Part model, mm, in its own coordinate system. A direction names the side the tool comes from. Round coordinates to 2 decimals unless told otherwise and drop trailing zeros. Loops run counter-clockwise (first coordinate to the right, second up) from the corner with the lowest first, then second, coordinate; pieces in that order, holes last. Notation, with made-up numbers: M 50.5,-34.75 L 98.5,-34.75 A14 cw 98.5,-20.75 Z; hole C -31.5,60.25 d4. An arc over 180 degrees is marked long. Put each result on its own line as item: value. Start each with the question number.
1) Slice it at B-B on z = 0. Give the cut face in (x, y).
2) Slice it at D-D on y = 34. Give the cut face in (x, z).
3) Probe line 1 along Y through (x, z) = (48.95, 9); line 2 along X through (y, z) = (42.5, 0); line 3 along Z through (x, y) = (21, 56). List the from-to ranges inside material, lowest first.
4) Slice it at A-A on y = 13.27. Give the cut face in (x, z), then the cut area to 3 significant figures.
5) Drop flat-ended pins along their axis: pin 1 Ø6.5 at (y, z) = (38.5, 9.5) entering from -X; pin 2 Ø8 at (x, y) = (-5.5, 7) entering from +Z. Give the stop position or say it passes through.
6) Pull direction X, two halves, no side cores. Call faces 4 (the flat face through (-1, 0, -2)), 5 (the flat face through (47, 38, 9)), 6 (the cylindrical face through (-47.464, 33.736, -0.325)): +X half, -X half, draft (parallel to the pull), parting line (faces both ways), or undercut.
7) Slice it at C-C on x = -46. Give the cut face in (y, z), then the cut area to 3 significant figures.
8) Which spindle directions (+Z, -Z, +X, -X, +Y, -Y) get a long thin tool onto all of the face, cutting with end or side? Do faces 1 (the flat face through (3.5, 10, 4.6)), 2 (the flat face through (50, 33, 4)), 3 (the flat face through (-2, 38, 5)). Say none if no direction does.
```python
from build123d import *

# Parameters (mm, degrees)
SKETCH1_W           = 100
SKETCH1_H           = 10
BOSS_EXTRUDE1_DEPTH = 66.54
CUT_EXTRUDE1_REACH  = 85.382
SKETCH2_R           = 1.5
LPATTERN1_COUNT     = 2
LPATTERN1_PITCH     = 92
SKETCH3_W           = 100
SKETCH3_H           = 10
CUT_EXTRUDE2_DEPTH  = 3
SKETCH4_W           = 3
SKETCH4_H           = 56.54
BOSS_EXTRUDE2_DEPTH = 8
CUT_EXTRUDE3_REACH  = 122.816
SKETCH5_R           = 1.5


with BuildPart() as part:
    # Sketch1 → Boss-Extrude1 (new body)
    with BuildSketch(Plane(origin=(0, 0, 0), x_dir=(1, 0, 0), z_dir=(0, 1, 0))):
        Rectangle(SKETCH1_W, SKETCH1_H)
    extrude(amount=BOSS_EXTRUDE1_DEPTH)

    # Sketch2 → Cut-Extrude1 (cut, up to next)
    with BuildSketch(Plane(origin=(0, 66.54, 0), x_dir=(1, 0, 0), z_dir=(0, 1, 0)), mode=Mode.PRIVATE) as cut_extrude1_sk1:
        with Locations(Location((-46, 0, 0), (0, 0, 270))):
            Circle(SKETCH2_R)
    cut_extrude1_tool1 = extrude(cut_extrude1_sk1.sketch, amount=-CUT_EXTRUDE1_REACH, mode=Mode.PRIVATE) & part.part
    cut_extrude1 = cut_extrude1_tool1.solids().sort_by_distance((-46, 66.54, 0))[0]
    add(cut_extrude1, mode=Mode.SUBTRACT)

    # LPattern1: Cut-Extrude1 ×2
    with Locations(*[(i * LPATTERN1_PITCH, 0, 0) for i in range(1, LPATTERN1_COUNT)]):
        add(cut_extrude1, mode=Mode.SUBTRACT)

    # Sketch3 → Cut-Extrude2 (cut)
    with BuildSketch(Plane.XY.offset(5)):
        with Locations((0, 5)):
            Rectangle(SKETCH3_W, SKETCH3_H)
    extrude(amount=-CUT_EXTRUDE2_DEPTH, mode=Mode.SUBTRACT)

    # Sketch4 → Boss-Extrude2 (add)
    with BuildSketch(Plane.XY.offset(5)):
        with Locations((48.5, 38.27)):
            Rectangle(SKETCH4_W, SKETCH4_H)
    extrude(amount=BOSS_EXTRUDE2_DEPTH)

    # Sketch5 → Cut-Extrude3 (cut, up to next)
    with BuildSketch(Plane(origin=(50, 0, 0), x_dir=(0, 0, -1), z_dir=(1, 0, 0)), mode=Mode.PRIVATE) as cut_extrude3_sk1:
        with Locations((-9, 58.27)):
            Circle(SKETCH5_R)
    cut_extrude3_tool1 = extrude(cut_extrude3_sk1.sketch, amount=-CUT_EXTRUDE3_REACH, mode=Mode.PRIVATE) & part.part
    # Sketch5 → Cut-Extrude3 (cut, up to next)
    with BuildSketch(Plane(origin=(50, 0, 0), x_dir=(0, 0, -1), z_dir=(1, 0, 0)), mode=Mode.PRIVATE) as cut_extrude3_sk2:
        with Locations((-9, 13.27)):
            Circle(SKETCH5_R)
    cut_extrude3_tool2 = extrude(cut_extrude3_sk2.sketch, amount=-CUT_EXTRUDE3_REACH, mode=Mode.PRIVATE) & part.part
    add(cut_extrude3_tool1.solids().sort_by_distance((50, 58.27, 9))[0], mode=Mode.SUBTRACT)
    add(cut_extrude3_tool2.solids().sort_by_distance((50, 13.27, 9))[0], mode=Mode.SUBTRACT)


solid = part.part
```
Recorded:
1. outline: M -50,0 L -47.5,0 L -47.5,66.54 L -50,66.54 Z; M -44.5,0 L 44.5,0 L 44.5,66.54 L -44.5,66.54 Z; M 47.5,0 L 50,0 L 50,66.54 L 47.5,66.54 Z
2. outline: M -50,-5 L 50,-5 L 50,13 L 47,13 L 47,5 L -50,5 Z; hole C -46,0 d3; hole C 46,0 d3
3. line 1: y = 10 to 11.77, 14.77 to 56.77, 59.77 to 66.54
3. line 2: x = -50 to -47.5, -44.5 to 44.5, 47.5 to 50
3. line 3: z = -5 to 5
4. outline: M -50,-5 L 50,-5 L 50,7.5 L 47,7.5 L 47,5 L -50,5 Z; M 47,10.5 L 50,10.5 L 50,13 L 47,13 Z; hole C -46,0 d3; hole C 46,0 d3
4. area: 1,000 mm2
5. pin 1: stops at x = 47
5. pin 2: stops at z = 5
6. face 4: draft
6. face 5: -X half
6. face 6: undercut
7. outline: M 0,-5 L 66.54,-5 L 66.54,-1.5 L 0,-1.5 Z; M 0,1.5 L 66.54,1.5 L 66.54,5 L 10,5 L 10,2 L 0,2 Z
7. area: 436 mm2
8. face 1: +Z, +X, -X, -Y
8. face 2: +Z, -Z, +X, +Y, -Y
8. face 3: +Z, -X, +Y, -Y
